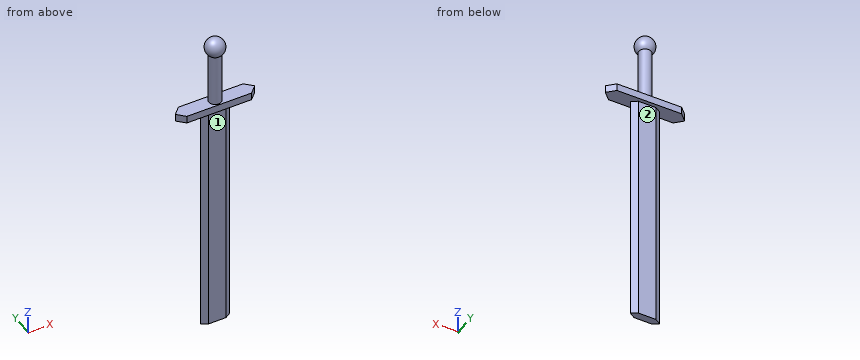
from build123d import *

# Parameters (mm, degrees)
F1_DEPTH    = 76.2
F2_W        = 38.1
F2_H        = 6.35
F3_DEPTH    = 3.175
F4_T1_DEPTH = 29.3032991577
F5_R        = 2.6614768155
F6_DEPTH    = 25.4
F10_DEPTH   = 25.4


# Not quite as in the source:
# - a fillet or chamfer that OpenCascade refuses, or shapes differently, is made with other operations: its cross-section is extruded or revolved along the edge and cut away or added


with BuildPart() as f1:
    # F0 (on Top) → F1 (new body)
    with BuildSketch(Plane.XY):
        Polygon((0, 1.5875), (-3.81, 1.5875), (-6.35, 0), (-3.81, -1.5875), (0, -1.5875), (3.81, -1.5875), (6.35, 0), (3.81, 1.5875), align=None)
    extrude(amount=F1_DEPTH)

    # F2 (on face) → F3 (join)
    with BuildSketch(Plane.XY.offset(76.2)):
        Rectangle(F2_W, F2_H)
    extrude(amount=F3_DEPTH)

    # F4: chamfer of 5.08 on 4 edges, made by hand

    # F4_s2 → F4_t1 (cut)
    with BuildSketch(Plane.XY.offset(63.1358504211)):
        Polygon((19.05, 1.905), (13.97, -3.175), (19.05, -3.175), align=None)
        Polygon((13.97, 3.175), (19.05, -1.905), (19.05, 3.175), align=None)
        Polygon((-19.05, 1.905), (-13.97, -3.175), (-19.05, -3.175), align=None)
        Polygon((-13.97, 3.175), (-19.05, -1.905), (-19.05, 3.175), align=None)
    extrude(amount=F4_T1_DEPTH, mode=Mode.SUBTRACT)

    # F5 (on face) → F6 (join)
    with BuildSketch(Plane.XY.offset(79.375)):
        Circle(F5_R)
    extrude(amount=F6_DEPTH)

    # F7 (on Front) → F9 (revolve)
    with BuildSketch(Plane.XZ):
        with BuildLine():
            Line((0, 108.979212298), (0, 100.7914969782))
            ThreePointArc((0, 100.7914969782), (4.0938576599, 104.8853546381), (0, 108.979212298))
        make_face()
    revolve(axis=Axis((0, 0, 105.8157756925), (0, 0, 1)))

    # F10 (add): a face of the model
    f10_faces = [f1.faces().sort_by_distance(p)[0] for p in [
        (0, 0, 0),
    ]]
    extrude(f10_faces, amount=F10_DEPTH)


solid = f1.part
Part model, mm, in its own coordinate system. Face numbers are marked on the shaded views. A direction names the side the tool comes from. Coordinates: 2 decimals unless noted, no trailing zeros. Order: outer loops, then holes, each group sorted by start corner. A loop starts at its lowest first (then second) coordinate and runs counter-clockwise, first axis right, second up. Notation, with made-up numbers: M 64,50 L 104,50 A22 cw 104,60 Z; hole C 27,-28 d3. An arc over 180 degrees is marked long. Use a Markdown table: item, result.
(1) Tool access for the marked faces 1 and 2: list every direction of +Z, -Z, +X, -X, +Y, -Y with a clear straight run to the whole face (end or side of a thin tool).
A:
| item | result |
|---|---|
| face 1 | -Z, +X, -X, -Y |
| face 2 | -Z, +X, -X, +Y |
(2) Cut at B-B on x = 0. Write the cut outline in (y, z) (1 decimal).
A:
| item | result |
|---|---|
| outline | M -3.2,76.2 L -1.6,76.2 L -1.6,-25.4 L 1.6,-25.4 L 1.6,76.2 L 3.2,76.2 L 3.2,79.4 L 2.7,79.4 L 2.7,101.8 A4.1 ccw long -2.7,101.8 L -2.7,79.4 L -3.2,79.4 Z |
(3) Probe L1, parallel to Y at x = 3, z = 51; L2, parallel to Z at x = -11, y = -3 (3 decimals); L3, parallel to X at y = 2.5, z = 76.5 (3 decimals). List the from-to ranges inside material, lowest first.
A:
| item | result |
|---|---|
| L1 | y = -1.59 to 1.59 |
| L2 | z = 76.2 to 79.375 |
| L3 | x = -14.645 to 14.645 |
(4) Cut at A-A on z = 70. Write the cut outline in (x, y), then the cut area to 3 significant figures.
A:
| item | result |
|---|---|
| outline | M -6.35,0 L -3.81,-1.59 L 3.81,-1.59 L 6.35,0 L 3.81,1.59 L -3.81,1.59 Z |
| area | 32.3 mm^2 |
(5) Cut at C-C on x = 9. Write the cut outline in (y, z) (3 decimals).
A:
| item | result |
|---|---|
| outline | M -3.175,76.2 L 3.175,76.2 L 3.175,79.375 L -3.175,79.375 Z |
(6) Flat gauge pins, fed straight in: pin 1 (2.5 mm diameter, centred on x = -1, z = 2, fed in from +Y); pin 2 (1 mm diameter, centred on x = -5, z = 78, fed in from -Y) (3 decimals); pin 3 (8.5 mm diameter, centred on x = -2, z = 16.5, fed in from -Y); pin 4 (3 mm diameter, centred on x = -1, y = -1, fed in from +Z). Where does each tip first touch, or does it go through?
A:
| item | result |
|---|---|
| pin 1 | stops at y = 1.59 |
| pin 2 | stops at y = -3.175 |
| pin 3 | stops at y = -1.59 |
| pin 4 | stops at z = 108.98 |
